Autodesk Inventor part; units mm, degrees
ref_plane "Work Plane1" through (-2, 0, 0) normal (1, 0, 0) x (0, 0, -1)
ref_plane "YZ Plane" through (0, 0, 0) normal (1, 0, 0) x (0, 1, 0)
ref_plane "XZ Plane" through (0, 0, 0) normal (0, 1, 0) x (-1, 0, 0)
sketch "Sketch1" plane through (0, 0, 0) normal (0, 0, 1) x (1, 0, 0)
  line L0 (0, 0) -> (0, 44)
  line L1 (-14.0215, 3) -> (-31, 3)
  arc A0 (-31, 3) -> (-40, 0) centre (-35, 0) ccw
  line L2 (-40, 0) -> (0, 0)
  line L3 (0, 44) -> (-1, 44)
  line L4 (-1, 44) -> (-9.1378, 6.928)
  arc A1 (-14.0215, 3) -> (-9.1378, 6.928) centre (-14.0215, 8) ccw
  point P0 (-10, 3)
  dimension "d0" = 44
  dimension "d1" = 5
  dimension "d2" = 3
  dimension "d3" = 1
  dimension "d4" = 35
  dimension "d5" = 10
  dimension "d18" = 5
revolve "Revolution1" add sketch "Sketch1" angle 360 about axis through (-40, 0, 0) along (1, 0, 0)
sketch "Sketch2" plane through (0, 0, 0) normal (1, 0, 0) x (0, 0, -1)
  line L0 (0, 0) -> (35, 0) construction
  circle A0 centre (35, 0) radius 1.65
  dimension "d7" = 3.3
  dimension "d8" = 35
extrude "Extrusion1" cut sketch "Sketch2" against normal through all
ref_plane "Work Plane1" through (-2, 0, 0) normal (1, 0, 0) x (0, 0, -1)
sketch "Sketch3" plane through (-2, 0, 0) normal (1, 0, 0) x (0, 0, -1)
  circle A0 centre (35, 0) radius 3
  circle A1 centre (35, 0) radius 1.65
  point P0 (0, 0)
  dimension "d12" = 6
extrude "Extrusion2" cut sketch "Sketch3" against normal through all contours A0 | A1
pattern_circular "Circular Pattern1" count 6 over 360 about axis through (-22.5107, 0, 0) along (1, 0, 0) of "Extrusion2", "Extrusion1"
properties part number "TrainingTarget"
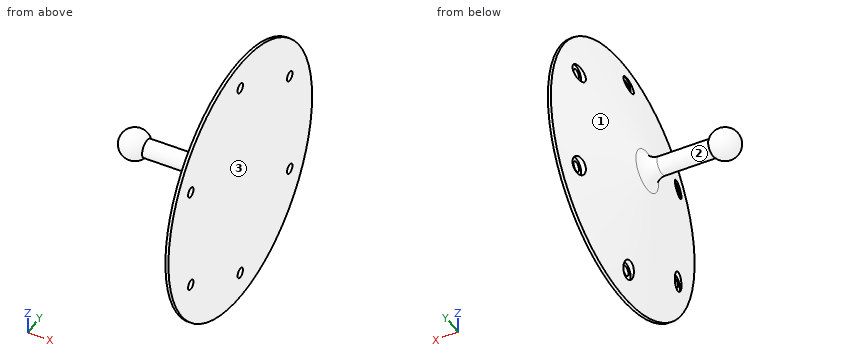
Can you work these out from the model? Positions are in its coordinate system, mm. Face numbers are marked on the shaded views. Coordinates: 2 decimals unless noted, no trailing zeros. Write each loop counter-clockwise with the first axis right and the second up, starting at its lowest first coordinate (ties: lowest second). Pieces come first, ordered by that corner, then holes. Notation, with made-up numbers: (-16, -33) -> (35, -33) arc R14 cw to (35, -16) -> close; hole circle Ø10 at (18.5, -4.75). An arc over 180 degrees is marked (long way). Write each question's results on one line, items separated by ' | '. Start each with the question number.
Q1. Imagine slicing it at B-B (y = 0). Write out the boundary of the cut face in (x, z).
Q2. Imagine slicing it at A-A (z = 0). Write out the boundary of the cut face in (x, y).
Q3. If I drill on probe 1 along X at (y, z) = (-2.5, 36); probe 2 along Y at (x, z) = (-2.6, 17.5); probe 3 along X at (y, z) = (-35.5, 21.5), over which ranges is the centre line in solid material (lowest first)?
Q4. We'd pull the mould along X, two halves only. Please class the marked faces 1, 2 and 3: +X half, -X half, draft (parallel to the pull), parting line (faces both ways), or undercut.
Q5. I'm going to push flat-ended pins straight in: pin 1 (10 mm diameter, centred on x = -24.5, y = -1.5, fed in from +Z); pin 2 (2.5 mm diameter, centred on y = -30.31, z = 17.5, fed in from -X); pin 3 (1.8 mm diameter, centred on y = 31.5, z = -18.5, fed in from -X); pin 4 (5 mm diameter, centred on y = -1, z = 33.5, fed in from -X). Where does each tip first touch, or does it pass through?
Taken from the geometry:
1) outline: (-31, -3) -> (-14.02, -3) arc R5 cw to (-9.14, -6.93) -> (-3.63, -32) -> (-2, -32) -> (-2, -33.35) -> (0, -33.35) -> (0, 33.35) -> (-2, 33.35) -> (-2, 32) -> (-3.63, 32) -> (-9.14, 6.93) arc R5 cw to (-14.02, 3) -> (-31, 3) arc R5 ccw (long way) to start; (-2.32, -38) -> (-1, -44) -> (0, -44) -> (0, -36.65) -> (-2, -36.65) -> (-2, -38) -> close; (-2.32, 38) -> (-2, 38) -> (-2, 36.65) -> (0, 36.65) -> (0, 44) -> (-1, 44) -> close
2) outline: (-31, -3) -> (-14.02, -3) arc R5 cw to (-9.14, -6.93) -> (-1, -44) -> (0, -44) -> (0, 44) -> (-1, 44) -> (-9.14, 6.93) arc R5 cw to (-14.02, 3) -> (-31, 3) arc R5 ccw (long way) to start
3) probe 1: x = -2 to 0 | probe 2: y = -27.31 to 27.31 | probe 3: x = -1.55 to 0
4) face 1: -X half | face 2: undercut | face 3: +X half
5) pin 1: stops at z = 3 | pin 2: passes through | pin 3: stops at x = -2 | pin 4: stops at x = -3.85
